```python
from build123d import *

# Parameters (mm, degrees)
SKETCH1_W           = 140
SKETCH1_H           = 40
BOSS_EXTRUDE1_DEPTH = 30
SKETCH2_W           = 137.2
SKETCH2_H           = 37.2
CUT_EXTRUDE1_DEPTH  = 28.4
SKETCH3_W           = 4.1
SKETCH3_H           = 4
CUT_EXTRUDE2_DEPTH  = 141
SKETCH4_W           = 2.05
SKETCH4_H           = 4
SKETCH4_W_2         = 4.1
CUT_EXTRUDE3_DEPTH  = 41


with BuildPart() as part:
    # Sketch1 → Boss-Extrude1 (new body)
    with BuildSketch(Plane(origin=(0, 0, 0), x_dir=(1, 0, 0), z_dir=(0, 1, 0))):
        Rectangle(SKETCH1_W, SKETCH1_H)
    extrude(amount=BOSS_EXTRUDE1_DEPTH)

    # Sketch2 → Cut-Extrude1 (cut)
    with BuildSketch(Plane.XZ):
        Rectangle(SKETCH2_W, SKETCH2_H)
    extrude(amount=-CUT_EXTRUDE1_DEPTH, mode=Mode.SUBTRACT)

    # Sketch3 → Cut-Extrude2 (cut, through all)
    with BuildSketch(Plane.ZY.offset(70)):
        with Locations((0, 6.25)):
            Rectangle(SKETCH3_W, SKETCH3_H)
    extrude(amount=-CUT_EXTRUDE2_DEPTH, mode=Mode.SUBTRACT)

    # Sketch4 → Cut-Extrude3 (cut, through all)
    with BuildSketch(Plane.XY.offset(20)):
        with Locations((-1.025, 6.25)):
            Rectangle(SKETCH4_W, SKETCH4_H)
        with Locations((-35, 6.25)):
            Rectangle(SKETCH4_W_2, SKETCH4_H)
    cut_extrude3 = extrude(amount=-CUT_EXTRUDE3_DEPTH, mode=Mode.SUBTRACT)

    # Mirror1: Cut-Extrude3 across plane
    add(cut_extrude3.mirror(Plane(origin=(0, 0, 0), x_dir=(0, 0, 1), z_dir=(1, 0, 0))), mode=Mode.SUBTRACT)


solid = part.part
```
Read the model definition and answer for the solid it produces. Units are mm, in the model's axes. A direction names the side the tool comes from. Give positions to 0.01 mm unless a question says otherwise; leave off trailing zeros. Write each loop counter-clockwise with the first axis right and the second up, starting at its lowest first coordinate (ties: lowest second). Pieces come first, ordered by that corner, then holes. Notation, with made-up numbers: (-11, 0.5) - (0, 0.5) arc R10 ccw to (0, 10.5) - close; hole circle Ø10 at (-36, 23.5). An arc over 180 degrees is marked (long way). Write item = value, one per line. Start each with the question number.
Item 1: Find section B-B (z = -13). Give the vertices of the cut face in (x, y), then the cut area to 3 significant figures.
Item 2: Find section A-A (y = 25). Give the vertices of the cut face in (x, z).
Item 3: Find section C-C (x = 50). Give the vertices of the cut face in (y, z).
Item 4: A tool of negligible diameter and unlimited length cuts with its end or side. For faces 4 (the flat face through (0, 0, -19)), 5 (the flat face through (-1, 14, -18.6)), from which of +Z, -Z, +X, -X, +Y, -Y can it reach the whole face along a straight path? Write none if from no direction.
Item 5: The mould has two halves that part along X. Classify faces 1 (the flat face through (-68.6, 14, 0)), 2 (the flat face through (70, 15, 0)), 3 (the flat face through (-1, 30, 0)): +X half, -X half, draft (parallel to the pull), parting line (faces both ways), or undercut.
Item 6: Find the intervals of material crossed by probe 1 along Z at (x, y) = (-53, 13); probe 2 along X at (y, z) = (6.5, 7.5); probe 3 along Y at (x, z) = (48, 17.5), in increasing order. Write a range as [from, to].
Item 7: This flat-tipped pin is pushed along its axis until it touches: P1, Ø1, axis at x = -31, z = 13, coming from the -Y side. Where does it stop, or does it pass through?
Response:
q1.outline = (-70, 0) - (-68.6, 0) - (-68.6, 28.4) - (68.6, 28.4) - (68.6, 0) - (70, 0) - (70, 30) - (-70, 30) - close
q1.area = 304 mm²
q2.outline = (-70, -20) - (70, -20) - (70, 20) - (-70, 20) - close; hole (-68.6, -18.6) - (68.6, -18.6) - (68.6, 18.6) - (-68.6, 18.6) - close
q3.outline = (0, -20) - (30, -20) - (30, 20) - (0, 20) - (0, 18.6) - (28.4, 18.6) - (28.4, -18.6) - (0, -18.6) - close
q4.face_4 = +Z, -Z, +X, -X, -Y
q4.face_5 = -Y
q5.face_1 = undercut
q5.face_2 = +X half
q5.face_3 = draft
q6.probe_1 = [-20, -18.6], [18.6, 20]
q6.probe_2 = [-70, -68.6], [68.6, 70]
q6.probe_3 = [28.4, 30]
q7.P1 = 28.4
